Verification items for the finished model (mm, model axes). Face numbers are marked on the shaded views. A direction names the side the tool comes from. Round coordinates to 2 decimals unless told otherwise and drop trailing zeros. Order: outer loops, then holes, each group sorted by start corner. A loop starts at its lowest first (then second) coordinate and runs counter-clockwise, first axis right, second up. Notation, with made-up numbers: M 9.25,10 L 62.25,10 A5 ccw 62.25,16 Z; hole C -4.5,-19 d10. An arc over 180 degrees is marked long. Write item = value, one per line. Start each with the question number.
Autodesk Inventor part; units mm, degrees
ref_plane "YZ Plane" through (0, 0, 0) normal (1, 0, 0) x (0, 1, 0)
ref_plane "XZ Plane" through (0, 0, 0) normal (0, 1, 0) x (-1, 0, 0)
ref_plane "XY Plane" through (0, 0, 0) normal (0, 0, 1) x (1, 0, 0)
sketch "Sketch1" plane through (0, 0, 0) normal (0, 0, 1) x (1, 0, 0)
  line L0 (16.4172, 2.5) -> (16.4172, 0)
  line L1 (-3.5828, 5.45) -> (-3.5828, 0)
  line L2 (-3.5828, 0) -> (16.4172, 0)
  line L3 (-4.3037, 0) -> (7.1102, 0)
  line L4 (-3.0328, 5.45) -> (-0.1414, 2.5586)
  line L5 (-3.5828, 5.45) -> (-3.0328, 5.45)
  line L6 (0, 2.5) -> (16.4172, 2.5)
  arc A0 (-0.1414, 2.5586) -> (0, 2.5) centre (0, 2.7) ccw
  line L7 (0, 2.5) -> (0, 0)
  point P0 (-0.0828, 2.5)
  dimension "d2" = 20
  dimension "d52" = 45
  dimension "d57" = 3.5
  dimension "d58" = 90
  dimension "d60" = 10.9
  dimension "d61" = 0.2
  dimension "d62" = 5
revolve "Revolution1" add sketch "Sketch1" angle 360 about axis through (-4.3037, 0, 0) along (1, 0, 0)
thread "Thread1"
chamfer "Chamfer1" distance 0.2 angle 45 1 edges at (16.4172, -2.5, 0)
sketch "Sketch2" plane through (-3.5828, 0, 0) normal (-1, 0, 0) x (0, 0, 1)
  circle A0 centre (0, 0) radius 2.25 construction
  circle A1 centre (0, 0) radius 1.575 construction
  line L0 (2.6829, 0) -> (-1.3062, 0) construction
  line L1 (0, 0) -> (1.364, 0.7875)
  line L2 (0, 0) -> (1.364, -0.7875)
  line L3 (1.364, 0.7875) -> (2.25, 0)
  line L4 (2.25, 0) -> (1.364, -0.7875)
  point P0 (0, 0)
  dimension "d17" = 4.5
  dimension "d18" = 3.15
  dimension "d19" = 30
  dimension "d20" = 30
  dimension "d21" = 83.262
extrude "Extrusion1" cut sketch "Sketch2" against normal blind 1.89
pattern_circular "Circular Pattern1" count 6 over 360 about axis through (-10, 0, 0) along (1, 0, 0) of "Extrusion1"
fillet "Fillet1" radius 0.5 11 edges at (-2.6378, 0.7875, 1.364) (-2.6378, -0.7875, 1.364) (-2.6378, -1.575, 0) (-2.6378, 0, 2.25) (-2.6378, 1.575, 0) (-2.6378, -0.7875, -1.364) (-2.6378, 0, -2.25) (-2.6378, -1.9486, 1.125) (-2.6378, -1.9486, -1.125) (-2.6378, 1.9486, -1.125) (-2.6378, 1.9486, 1.125)
equation "\"d2\" = l_"
equation "\"d52\" = 0.5 * headAngle"
equation "\"d60\" = dk"
equation "\"d61\" = r"
equation "\"d62\" = d_"
equation "\"d12\" = thredlenght"
equation "\"d17\" = A_"
equation "\"d18\" = 0.7 * A_"
equation "\"d22\" = t"
equation "\"d27\" = 0.1 * d_"
equation "\"p\" = 0.5"
equation "\"dk\" = 10.9"
equation "\"d_\" = 5"
equation "\"k\" = 3.5"
equation "\"r\" = 0.2"
equation "\"A_\" = 4.5"
equation "\"t\" = 1.89"
equation "\"l_\" = 20"
equation "\"lg\" = r + k"
equation "\"shldr\" = p"
equation "\"headAngle\" = 90deg"
equation "\"d53_Copy\" = 1.938"
equation "\"thredlenght\" = l_ - lg"
properties part number "Countersunk head screw ISO 14582 - M5x20-10.9" material "Steel"
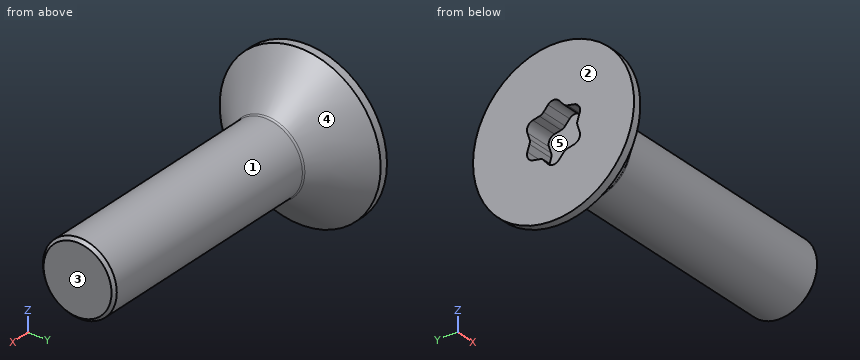
1) Cross-section at B-B, the plane x = 3.25. Enter the section's corners in (y, z), then the cut area to 3 significant figures.
2) Scan lines: probe 1 along X at (y, z) = (1.5, -0.5); probe 2 along Z at (x, y) = (15.5, -1.25); probe 3 along X at (y, z) = (-3.25, -3). Record each from-to range of solid material in increasing order.
3) Gauge pin test, flat ends, axial feed: P1, Ø6, axis at x = 1, y = 3, coming from the -Z side; P2, Ø3, axis at x = -0.5, z = -4, coming from the +Y side; P3, Ø2, axis at x = 13, z = 4.5, coming from the +Y side; P4, Ø6, axis at x = 4.5, y = 2.5, coming from the -Z side. Record the tip position at first contact, or that the pin passes through.
4) Cross-section at A-A, the plane y = 0. Enter the section's corners in (x, z).
5) Access from +Z, -Z, +X, -X, +Y, -Y to the whole of each face (thin tool, end or side, straight path). Record for the marked faces 1 and 2.
6) Release check for a two-part mould opening along Y. For the marked faces 3, 4 and 5 record: pulls with the +Y half, pulls with the -Y half, needs draft (parallel to the pull), parting line crosses it, or undercut.
7) Cross-section at C-C, the plane x = -1.25. Enter the section's corners in (y, z), then the cut area to 3 significant figures.
Geometry results:
q1.outline = C 0,0 d5
q1.area = 19.6 mm^2
q2.probe_1 = -1.69 to 16.42
q2.probe_2 = -2.17 to 2.17
q2.probe_3 = -3.58 to -2.01
q3.P1 = -3.76
q3.P2 = 2.71
q3.P3 = through
q3.P4 = -2.5
q4.outline = M -3.58,-5.45 L -3.03,-5.45 L -0.14,-2.56 A0.2 cw 0,-2.5 L 16.22,-2.5 L 16.42,-2.3 L 16.42,2.3 L 16.22,2.5 L 0,2.5 A0.2 cw -0.14,2.56 L -3.03,5.45 L -3.58,5.45 L -3.58,2 L -1.69,2 L -1.69,-2 L -3.58,-2 Z
q5.face_1 = +X
q5.face_2 = +Z, -Z, -X, +Y, -Y
q6.face_3 = needs draft
q6.face_4 = parting line crosses it
q6.face_5 = undercut
q7.outline = C 0,0 d7.33
q7.area = 42.2 mm^2
